from build123d import *

# Parameters (mm, degrees)
SKETCH1_R           = 3.175
BOSS_EXTRUDE1_DEPTH = 9.525
SKETCH3_R           = 2.54
CUT_EXTRUDE1_DEPTH  = 12.7
CUT_EXTRUDE2_REACH  = 865.776
SKETCH4_R           = 2.54
FILLET1_R           = 3.175
SKETCH5_R           = 12.7
CUT_EXTRUDE3_DEPTH  = 881.013791313


with BuildPart() as part:
    # Sketch1 → Boss-Extrude1 (new body)
    with BuildSketch(Plane.XY):
        with BuildLine():
            Line((-169.8874175, 850.687119625), (-169.8874175, 837.987119625))
            ThreePointArc((-169.8874175, 837.987119625), (-159.2194175, 827.319119625), (-169.8874175, 816.651119625))
            Line((-169.8874175, 816.651119625), (-169.8874175, 803.951119625))
            Line((-169.8874175, 803.951119625), (-150.8374175, 803.951119625))
            Line((-150.8374175, 803.951119625), (-133.8194175, 833.943095553))
            Line((-133.8194175, 833.943095553), (-133.8194175, 835.975095553))
            ThreePointArc((-133.8194175, 835.975095553), (-146.5194175, 848.675095553), (-133.8194175, 861.375095553))
            Line((-133.8194175, 861.375095553), (-133.8194175, 863.407095553))
            Line((-133.8194175, 863.407095553), (-152.8694175, 863.407095553))
            Line((-152.8694175, 863.407095553), (-169.8874175, 850.687119625))
        make_face()
        with Locations(Location((-153.108454604, 853.862119625, 0), (0, 0, 180))):
            Circle(SKETCH1_R, mode=Mode.SUBTRACT)
        with BuildLine():
            Line((-150.93222253, 816.651119625), (-142.409287823, 831.671665669))
            ThreePointArc((-142.409287823, 831.671665669), (-146.401670459, 834.371620085), (-149.588680975, 837.987119625))
            Line((-149.588680975, 837.987119625), (-156.628228233, 837.987119625))
            ThreePointArc((-156.628228233, 837.987119625), (-152.8694175, 827.319119625), (-156.628228233, 816.651119625))
            Line((-156.628228233, 816.651119625), (-150.93222253, 816.651119625))
        make_face(mode=Mode.SUBTRACT)
    extrude(amount=BOSS_EXTRUDE1_DEPTH)

    # Sketch3 → Cut-Extrude1 (cut)
    with BuildSketch(Plane.ZY.offset(169.8874175)):
        with Locations((4.7625, 845.607119625)):
            Circle(SKETCH3_R)
        with Locations((4.7625, 809.031119625)):
            Circle(SKETCH3_R)
    extrude(amount=-CUT_EXTRUDE1_DEPTH, mode=Mode.SUBTRACT)

    # Sketch4 → Cut-Extrude2 (cut, up to next)
    with BuildSketch(Plane.ZY.offset(157.1874175), mode=Mode.PRIVATE) as cut_extrude2_sk1:
        with Locations((4.7625, 809.031119625)):
            Circle(SKETCH4_R)
    cut_extrude2_tool1 = extrude(cut_extrude2_sk1.sketch, amount=-CUT_EXTRUDE2_REACH, mode=Mode.PRIVATE) & part.part
    add(cut_extrude2_tool1.solids().sort_by_distance((-157.187417, 809.03112, 4.7625))[0], mode=Mode.SUBTRACT)

    # Fillet1
    # the kernel refuses this fillet: 3.175 mm, written as the material it adds along each edge
    with BuildSketch(Plane(origin=(-150.93222253, 816.651119625, 0), x_dir=(0.4935074111606293, 0.8697415910082337, 0), z_dir=(0, 0, 1))) as fillet1_piece_1:
        with BuildLine():
            CenterArc((FILLET1_R * 0.582348359646, FILLET1_R), FILLET1_R, 209.571375415, 60.428624585)
            Line((-FILLET1_R * 0.287393231362, FILLET1_R * 0.506492588839), (0, 0))
            Line((0, 0), (FILLET1_R * 0.582348359646, 0))
        make_face()
    extrude(amount=9.525)
    with BuildSketch(Plane(origin=(-149.588680975, 837.987119625, 0), x_dir=(0.5928517761937993, -0.8053115989875331, 0), z_dir=(0, 0, 1))) as fillet1_piece_2:
        with BuildLine():
            CenterArc((1.606983899, -3.172592716), FILLET1_R, 92.231294299, 51.409064566)
            Line((-0.949880428, -1.290288327), (0, 0))
            ThreePointArc((0, 0), (0.741684876, -0.014443703), (1.483369753, 0))
        make_face()
    extrude(amount=9.525)
    with BuildSketch(Plane(origin=(-156.628228233, 837.987119625, 0), x_dir=(1, 0, 0), z_dir=(0, 0, 1))) as fillet1_piece_3:
        with BuildLine():
            CenterArc((5.49213602, -3.175), FILLET1_R, 90, 111.781571646)
            ThreePointArc((2.543814434, -4.353144654), (1.434014336, -2.081843008), (0, 0))
            Line((0, 0), (5.49213602, 0))
        make_face()
    extrude(amount=9.525)
    with BuildSketch(Plane(origin=(-156.628228233, 816.651119625, 0), x_dir=(0.5045338460547648, 0.8633919145933595, 0), z_dir=(0, 0, 1))) as fillet1_piece_4:
        with BuildLine():
            CenterArc((5.512237838, -3.139970872), FILLET1_R, 98.518841269, 111.781571646)
            Line((2.770968509, -4.741865834), (0, 0))
            ThreePointArc((0, 0), (2.520955189, -0.187756124), (5.041910378, 0))
        make_face()
    extrude(amount=9.525)
    with BuildSketch(Plane(origin=(-142.409287823, 831.671665669, 0), x_dir=(-0.49350741116063396, -0.869741591008231, 0), z_dir=(0, 0, 1))) as fillet1_piece_5:
        with BuildLine():
            CenterArc((3.082586278, -3.175), FILLET1_R, 90, 84.177526613)
            ThreePointArc((-0.07603388, -2.852907312), (0.015483213, -1.427879508), (0, 0))
            Line((0, 0), (3.082586278, 0))
        make_face()
    extrude(amount=9.525)
    # the kernel refuses this fillet: 3.175 mm, written as the material it takes off along each edge
    with BuildSketch(Plane(origin=(-152.8694175, 863.407095553, -2.638608517), x_dir=(-0.80098222360548, -0.5986881303884525, 0), z_dir=(0, 0, 1))) as fillet1_2_piece_1:
        with BuildLine():
            CenterArc((FILLET1_R * 0.332423120307, FILLET1_R), FILLET1_R, 233.22400043, 36.77599957)
            Line((-FILLET1_R * 0.266265010081, FILLET1_R * 0.199017776395), (0, 0))
            Line((0, 0), (FILLET1_R * 0.332423120307, 0))
        make_face()
    extrude(amount=14.802217035, mode=Mode.SUBTRACT)
    with BuildSketch(Plane(origin=(-150.8374175, 803.951119625, -4.622390105), x_dir=(-1, 0, 0), z_dir=(0, 0, 1))) as fillet1_2_piece_2:
        with BuildLine():
            CenterArc((FILLET1_R * 0.582348359646, -FILLET1_R), FILLET1_R, 90, 60.428624585)
            Line((-FILLET1_R * 0.287393231362, -FILLET1_R * 0.506492588839), (0, 0))
            Line((0, 0), (FILLET1_R * 0.582348359646, 0))
        make_face()
    extrude(amount=18.769780209, mode=Mode.SUBTRACT)

    # Sketch5 → Cut-Extrude3 (cut, through all)
    with BuildSketch(Plane(origin=(0, 0, 0), x_dir=(-1, 0, 0), z_dir=(0, 0, -1))):
        with Locations((169.8874175, 827.319119625)):
            Circle(SKETCH5_R)
    extrude(amount=-CUT_EXTRUDE3_DEPTH, mode=Mode.SUBTRACT)


solid = part.part
For this review, take the finished solid that the model builds, in its own axes (mm). A direction names the side the tool comes from. Give positions to 0.01 mm unless a question says otherwise; leave off trailing zeros. Loops run counter-clockwise (first coordinate to the right, second up) from the corner with the lowest first, then second, coordinate; pieces in that order, holes last.
Item 1: Take a section at D-D, the plane x = -141. State the section outline as (y, z) points (3 decimals), and give its area (3 significant figures).
Item 2: Tool access review of faces 1 (the flat face through (-157.187, 846, 5)), 2 (the cylindrical face through (-152.87, 827.41, 4.7)), 3 (the cylindrical face through (-152.8, 863.25, 4.7)): name each direction out of +Z, -Z, +X, -X, +Y, -Y from which nothing blocks a thin tool from reaching the whole face with its end or side.
Item 3: Take a section at B-B, the plane x = -164.5. State the section outline as (y, z) points (1 decimal).
Item 4: Take a section at C-C, the plane y = 824.5. State the section outline as (x, z) points (3 decimals).
Item 5: Take a section at A-A, the plane z = 4. Give the number of separate pieces and of enclosed holes in the cut face, and give its area (3 significant figures).
Item 6: Insertion check: pin 1 (3 mm diameter, centred on x = -166, z = 8, fed in from +Y); pin 2 (12 mm diameter, centred on x = -145, y = 829, fed in from +Z) (3 decimals); pin 3 (4.5 mm diameter, centred on y = 845.61, z = 4.76, fed in from -X); pin 4 (4 mm diameter, centred on y = 814.5, z = 4.5, fed in from +X). Each pin has a flat end and moves straight along its axis. Give the tip position at first contact, or say it passes through.
Item 7: For line 1 along Y through (x, z) = (-152, 1.5); line 2 along X through (y, z) = (853, 5.5); line 3 along X through (y, z) = (821, 7), list the stretches that pass through material, from the lowest coordinate up.
Item 8: Draft analysis for pull direction X (two halves, no side actions). For faces 4 (the cylindrical face through (-146.516, 848.396, 4.696)), 5 (the cylindrical face through (-158.36, 811.55, 4.43)), 6 (the cylindrical face through (-153.748, 836.617, 4.696)), 7 (the flat face through (-161.688, 856.816, 4.696)), state which applies: +X half, -X half, draft (parallel to the pull), parting line (faces both ways), or undercut.
Calculated:
1. outline: (821.288, 0) - (838.2, 0) - (838.2, 9.525) - (821.288, 9.525) - close; (859.15, 0) - (863.407, 0) - (863.407, 9.525) - (859.15, 9.525) - close
1. area: 202 mm2
2. face 1: -X
2. face 2: +Z, -Z
2. face 3: +Z, -Z, -X, +Y
3. outline: (804, 0) - (815.8, 0) - (815.8, 9.5) - (804, 9.5) - close; (838.8, 0) - (854.7, 0) - (854.7, 9.5) - (838.8, 9.5) - close; hole circle Ø5.1 at (809, 4.8); hole circle Ø5.1 at (845.6, 4.8)
4. outline: (-157.504, 0) - (-153.105, 0) - (-153.105, 9.525) - (-157.504, 9.525) - close; (-146.479, 0) - (-139.178, 0) - (-139.178, 9.525) - (-146.479, 9.525) - close
5. separate pieces: 2
5. enclosed holes: 2
5. area: 931 mm2
6. pin 1: stops at y = 854.71
6. pin 2: stops at z = 9.525
6. pin 3: stops at x = -157.19
6. pin 4: stops at x = -143.72
7. line 1: y = 804.03 to 816.77, 837.87 to 850.89, 856.84 to 863.4
7. line 2: x = -166.79 to -156.16, -150.05 to -145.76
7. line 3: x = -158.87 to -154.09, -148.46 to -141.16
8. face 4: +X half
8. face 5: draft
8. face 6: undercut
8. face 7: -X half
